Autodesk Fusion 360 part; units mm, degrees
sketch "Szkic1" plane through (0, 0, 0) normal (0, 0, 1) x (1, 0, 0)
  line L0 (0, 0) -> (75, 0)
  line L1 (75, 0) -> (75, 40)
  line L2 (75, 40) -> (0, 40)
  line L3 (0, 40) -> (0, 0)
  dimension "d1" = 75
  dimension "d2" = 40
extrude "Wyciągnięcie proste1" add sketch "Szkic1" along normal blind 20 makes body 1
shell "Skorupa1" thickness 2 removed faces 1 at (25, 26.6667, 20) on bodies 1
extrude "Wyciągnięcie proste2" add 1 faces at (25, 26.6667, 0) along direction (0, 0, 1) blind 5 on bodies 1 bodies 1
copy_body "Bryła->Komponent1" bodies 1 removing the originals makes body 2 in component "koszyk"
component "koszyk" placed x (1, 0, 0) y (0, 1, 0) z (0, 0, 1) at (0, 0, 0)
Here's how the part is built. I have some questions about the finished solid (model axes, mm). A direction names the side the tool comes from. Coordinates: 2 decimals unless noted, no trailing zeros. Write each loop counter-clockwise with the first axis right and the second up, starting at its lowest first coordinate (ties: lowest second). Pieces come first, ordered by that corner, then holes.
Item 1: I want a section at B-B on x = 10. Write out the boundary of the cut face in (y, z), and give its area (3 significant figures).
Item 2: Will this pin go through, and if not, where does the flat tip stop? pin 1 (3 mm diameter, centred on x = 18, y = 6, fed in from +Z).
Item 3: I want a section at C-C on y = 7.5. Write out the boundary of the cut face in (x, z), and give its area (3 significant figures).
Item 4: I want a section at A-A on z = 6.25. Write out the boundary of the cut face in (x, y), and give its area (3 significant figures).
Item 5: On a 3-axis mill with a long thin cutter (end or side, diameter ignored), from which of +Z, -Z, +X, -X, +Y, -Y can I reach the whole of each face in a straight line? I mean faces 5 (the flat face through (37, 0, 10)), 6 (the flat face through (2, 20, 12)). Say none if no direction works.
Item 6: If we mould it in two halves opening along X, with no side actions, what happens to faces 1 (the flat face through (37, 20, 0)), 2 (the flat face through (0, 20, 10)), 3 (the flat face through (37, 2, 12)), 4 (the flat face through (75, 20, 10))? For each: +X half, -X half, draft (parallel to the pull), parting line (faces both ways), or undercut.
Item 7: If I drill on line 1 (Y direction, x = 40, z = 6.75); line 2 (X direction, y = 28, z = 7.75); line 3 (Z direction, x = 20, y = 30), over which ranges is the centre line in solid material (lowest first)?
Findings below:
1. outline: (0, 0) - (40, 0) - (40, 20) - (38, 20) - (38, 5) - (2, 5) - (2, 20) - (0, 20) - close
1. area: 260 mm2
2. pin 1: stops at z = 5
3. outline: (0, 0) - (75, 0) - (75, 20) - (73, 20) - (73, 5) - (2, 5) - (2, 20) - (0, 20) - close
3. area: 435 mm2
4. outline: (0, 0) - (75, 0) - (75, 40) - (0, 40) - close; hole (2, 2) - (73, 2) - (73, 38) - (2, 38) - close
4. area: 444 mm2
5. face 5: +Z, -Z, +X, -X, -Y
5. face 6: +Z
6. face 1: draft
6. face 2: -X half
6. face 3: undercut
6. face 4: +X half
7. line 1: y = 0 to 2, 38 to 40
7. line 2: x = 0 to 2, 73 to 75
7. line 3: z = 0 to 5
